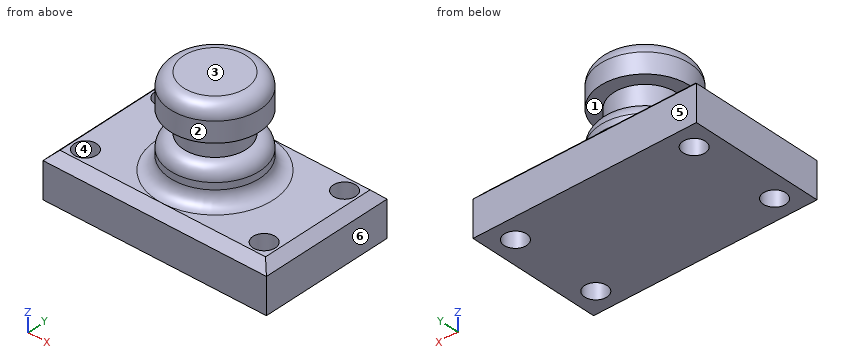
from build123d import *

# Parameters (mm, degrees)
F0_W     = 127
F0_H     = 76.2
F1_DEPTH = 12.7
F2_R     = 6.35
F3_DEPTH = 38.1
F4_W     = 25.4
F4_H     = 50.8
F6_W     = 16.0364900438
F6_H     = 12.7
F8_SIZE  = 5.08
F9_R     = 7.61999


# Not quite as in the source:
# - a fillet or chamfer is up to 0.001 mm smaller than in the source, because OpenCascade refuses the exact size


with BuildPart() as f1:
    # F0 (on Top) → F1 (new body, symmetric)
    with BuildSketch(Plane.XY):
        Rectangle(F0_W, F0_H)
    extrude(amount=F1_DEPTH, both=True)

    # F2 (on face) → F3 (cut)
    with BuildSketch(Plane.XY.offset(12.7)):
        with Locations((-50.8, 25.4)):
            Circle(F2_R)
        with Locations((50.8, 25.4)):
            Circle(F2_R)
        with Locations((50.8, -25.4)):
            Circle(F2_R)
        with Locations((-50.8, -25.4)):
            Circle(F2_R)
    extrude(amount=-F3_DEPTH, mode=Mode.SUBTRACT)

    # F4 (on Front) → F5 (revolve)
    with BuildSketch(Plane.XZ):
        with Locations((-12.7, 38.1)):
            Rectangle(F4_W, F4_H)
    revolve(axis=Axis((0, 0, 38.1), (0, 0, 1)))

    # F6 (on Front) → F7 (revolve, cut)
    with BuildSketch(Plane.XZ):
        with Locations((-25.7982450219, 38.1)):
            Rectangle(F6_W, F6_H)
    revolve(axis=Axis((0, 0, 63.5), (0, 0, -1)), mode=Mode.SUBTRACT)

    # F8
    f8_edges = [f1.edges().sort_by_distance(p)[0] for p in [
        (0, -38.1, 12.7),
        (-63.5, 0, 12.7),
        (0, 38.1, 12.7),
        (63.5, 0, 12.7),
    ]]
    chamfer(f8_edges, length=F8_SIZE)

    # F9 (radius 7.62 in the source; OpenCascade refuses exactly that, so slightly less here)
    f9_edges = [f1.edges().sort_by_distance(p)[0] for p in [
        (25.4, 0, 12.7),
        (25.4, 0, 31.75),
        (25.4, 0, 63.5),
    ]]
    fillet(f9_edges, radius=F9_R)


solid = f1.part
Verification items for the finished model (mm, model axes). Face numbers are marked on the shaded views. A direction names the side the tool comes from. Round coordinates to 2 decimals unless told otherwise and drop trailing zeros. Write each loop counter-clockwise with the first axis right and the second up, starting at its lowest first coordinate (ties: lowest second). Pieces come first, ordered by that corner, then holes.
(1) Material ranges on line 1 (X direction, y = 25, z = -1); line 2 (Y direction, x = -50.8, z = 4.75); line 3 (X direction, y = 23, z = -2.5), recorded low to high.
Returned:
line 1: x = -63.5 to -57.14, -44.46 to 44.46, 57.14 to 63.5
line 2: y = -38.1 to -31.75, -19.05 to 19.05, 31.75 to 38.1
line 3: x = -63.5 to -56.68, -44.92 to 44.92, 56.68 to 63.5
(2) Section check A-A (x = 50.8). Enter the section's corners in (y, z), plus the area to 3 significant figures.
Returned:
outline: (-38.1, -12.7) - (-31.75, -12.7) - (-31.75, 12.7) - (-33.02, 12.7) - (-38.1, 7.62) - close; (-19.05, -12.7) - (19.05, -12.7) - (19.05, 12.7) - (-19.05, 12.7) - close; (31.75, -12.7) - (38.1, -12.7) - (38.1, 7.62) - (33.02, 12.7) - (31.75, 12.7) - close
area: 1,260 mm2
(3) Access from +Z, -Z, +X, -X, +Y, -Y to the whole of each face (thin tool, end or side, straight path). Record for the marked faces 1, 2 and 3.
Returned:
face 1: none
face 2: +Z
face 3: +Z, +X, -X, +Y, -Y
(4) Mould release check, pull along Y, two halves, no side actions. Record for the marked faces 4, 5 and 6: pulls with the +Y half, pulls with the -Y half, needs draft (parallel to the pull), parting line crosses it, or undercut.
Returned:
face 4: undercut
face 5: pulls with the +Y half
face 6: needs draft
(5) Section check D-D (z = 33.5). Enter the section's corners in (x, y), plus the area to 3 significant figures.
Returned:
outline: circle Ø35.56 at (0, 0)
area: 993 mm2
(6) Depth check by flat-ended pin: pin 1 Ø5 at (y, z) = (11, 28) entering from +X; pin 2 Ø12 at (x, z) = (-16, 21.5) entering from +Y; pin 3 Ø14.5 at (x, y) = (50.8, -25.4) entering from +Z; pin 4 Ø11.5 at (x, y) = (50.8, 25.4) entering from -Z. Enter the tip coordinate at first touch or a pass-through.
Returned:
pin 1: stops at x = 23.35
pin 2: stops at y = 23.35
pin 3: stops at z = 12.7
pin 4: passes through
